from build123d import *

# Parameters (mm, degrees)
F1_DEPTH = 22.86
F2_R     = 9.525
F3_DEPTH = 25.4
F4_R     = 6.35
F5_R     = 15.875


with BuildPart() as f1:
    # F0 (on Front) → F1 (new body, symmetric)
    with BuildSketch(Plane.XZ):
        with BuildLine():
            Line((382.5875, -381), (471.4875, -381))
            Line((471.4875, -381), (471.4875, -368.3))
            Line((471.4875, -368.3), (395.2875, -368.3))
            Line((395.2875, -368.3), (395.2875, 0))
            ThreePointArc((395.2875, 0), (0, 395.2875), (-395.2875, 0))
            Line((-395.2875, 0), (-395.2875, -368.3))
            Line((-395.2875, -368.3), (-471.4875, -368.3))
            Line((-471.4875, -368.3), (-471.4875, -381))
            Line((-471.4875, -381), (-382.5875, -381))
            Line((-382.5875, -381), (-382.5875, 0))
            ThreePointArc((-382.5875, 0), (0, 382.5875), (382.5875, 0))
            Line((382.5875, 0), (382.5875, -381))
        make_face()
    extrude(amount=F1_DEPTH, both=True)

    # F2 (on face) → F3 (cut)
    with BuildSketch(Plane(origin=(0, 0, -381), x_dir=(1, 0, 0), z_dir=(0, 0, -1))):
        with Locations((-439.7375, 0)):
            Circle(F2_R)
        with Locations((439.7375, 0)):
            Circle(F2_R)
    extrude(amount=-F3_DEPTH, mode=Mode.SUBTRACT)

    # F4
    f4_edges = [f1.edges().sort_by_distance(p)[0] for p in [
        (-395.2875, 0, -368.3),
        (395.2875, 0, -368.3),
    ]]
    fillet(f4_edges, radius=F4_R)

    # F5
    f5_edges = [f1.edges().sort_by_distance(p)[0] for p in [
        (-382.5875, 0, -381),
        (382.5875, 0, -381),
    ]]
    fillet(f5_edges, radius=F5_R)


solid = f1.part
For this review, take the finished solid that the model builds, in its own axes (mm). A direction names the side the tool comes from. Give positions to 0.01 mm unless a question says otherwise; leave off trailing zeros. Order: outer loops, then holes, each group sorted by start corner. A loop starts at its lowest first (then second) coordinate and runs counter-clockwise, first axis right, second up. Notation, with made-up numbers: M -14.75,60 L 25.25,60 A22 cw 25.25,73 Z; hole C 16.5,53.25 d8. An arc over 180 degrees is marked long. Answer in a Markdown table with one row per item. Add a question column.
(1) Wall thickness on probe 1 along X at (y, z) = (-7.5, -82); probe 2 along X at (y, z) = (0, -378); probe 3 along X at (y, z) = (0, -375): over which ranges is each line inside the solid? List them lowest first. Write a range as [from, to].
(2) For pin 1 (25 mm diameter, centred on x = -439.74, y = 0, fed in from -Z); pin 2 (6 mm diameter, centred on y = 8, z = 47.5, fed in from +X); pin 3 (1 mm diameter, centred on y = -9, z = -242.5, fed in from -X); pin 4 (3 mm diameter, centred on y = -15.5, z = 260.5, fed in from -X), all flat-tipped, find the tip position at first contact; note any pin that passes through.
(3) Consider section B-B on y = 0. Give the number of separate pieces and of enclosed holes in the cut face, and give its area (3 significant figures).
(4) Consider section D-D on z = 331. State the section outline as (x, y) points.
(5) For faces 1 (the face through (-428, 0, -368.3)), 2 (the face through (395.288, 0, -184)), 3 (the face through (-382.588, 0, -185)), list the 3-axis set-ups (+Z, -Z, +X, -X, +Y, -Y) from which the entire face can be reached by the end or side of a thin tool; tool diameter is ignored.
(6) Mouldability with a two-part tool opening along X and no side actions: class faces 4 (the face through (429, 0, -368.3)), 5 (the face through (382.588, 0, -180)), 6 (the face through (-395.288, 0, -178)) as +X half, -X half, draft (parallel to the pull), parting line (faces both ways), or undercut.
(7) Consider section C-C on x = 0. State the section outline as (y, z) points, and give its area (3 significant figures).
(8) Consider section A-A on z = -156.5. State the section outline as (x, y) points, and give its area (3 significant figures).
Evaluation:
| question | item | result |
|---|---|---|
| 1 | probe 1 | x = [-395.29, -382.59], [382.59, 395.29] |
| 1 | probe 2 | x = [-471.49, -449.26], [-430.21, -389.18], [389.18, 430.21], [449.26, 471.49] |
| 1 | probe 3 | x = [-471.49, -449.26], [-430.21, -386.03], [386.03, 430.21], [449.26, 471.49] |
| 2 | pin 1 | stops at z = -381 |
| 2 | pin 2 | stops at x = 392.77 |
| 2 | pin 3 | stops at x = -395.29 |
| 2 | pin 4 | stops at x = -298.62 |
| 3 | separate pieces | 3 |
| 3 | enclosed holes | 0 |
| 3 | area | 26,600 mm^2 |
| 4 | outline | M -216.08,-22.86 L -191.87,-22.86 L -191.87,22.86 L -216.08,22.86 Z; M 191.87,-22.86 L 216.08,-22.86 L 216.08,22.86 L 191.87,22.86 Z |
| 5 | face 1 | +Z, -X, +Y, -Y |
| 5 | face 2 | +Z, +X, +Y, -Y |
| 5 | face 3 | -Z, +Y, -Y |
| 6 | face 4 | draft |
| 6 | face 5 | undercut |
| 6 | face 6 | -X half |
| 7 | outline | M -22.86,382.59 L 22.86,382.59 L 22.86,395.29 L -22.86,395.29 Z |
| 7 | area | 581 mm^2 |
| 8 | outline | M -395.29,-22.86 L -382.59,-22.86 L -382.59,22.86 L -395.29,22.86 Z; M 382.59,-22.86 L 395.29,-22.86 L 395.29,22.86 L 382.59,22.86 Z |
| 8 | area | 1,160 mm^2 |
